Could you check a few things on this model? Use its own coordinates, in mm. A direction names the side the tool comes from. Coordinates: 2 decimals unless noted, no trailing zeros. Write each loop counter-clockwise with the first axis right and the second up, starting at its lowest first coordinate (ties: lowest second). Pieces come first, ordered by that corner, then holes. Notation, with made-up numbers: M 55,-15.75 L 102,-15.75 A21 cw 102,12.25 Z; hole C 29,8 d7. An arc over 180 degrees is marked long. Write item = value, one per line.
```python
from build123d import *

# Parameters (mm, degrees)
IZIM2_R                     = 5
Y_KSEKLIK_EKSTR_ZYON2_DEPTH = 21.5
IZIM2_5_R                   = 7.5
IZIM2_5_R_2                 = 5
Y_KSEKLIK_EKSTR_ZYON3_DEPTH = 16.5
IZIM18_R                    = 10
Y_KSEKLIK_EKSTR_ZYON6_DEPTH = 7.5
IZIM3_R                     = 7.5
Y_KSEKLIK_EKSTR_ZYON4_DEPTH = 50
S_P_R4_PROFILE_R            = 7.5
IZIM42_R                    = 5
KES_EKSTR_ZYON5_DEPTH       = 10
IZIM43_R                    = 5
Y_KSEKLIK_EKSTR_ZYON7_DEPTH = 15
IZIM44_R                    = 2.5
Y_KSEKLIK_EKSTR_ZYON8_DEPTH = 15


with BuildPart() as part:
    # izim2 → Y_kseklik-Ekstr_zyon2 (new, symmetric)
    with BuildSketch(Plane(origin=(0, 0, 0), x_dir=(1, 0, 0), z_dir=(0, 1, 0))):
        with Locations(Location((0, 0, 0), (0, 0, 270))):
            Circle(IZIM2_R)
    extrude(amount=Y_KSEKLIK_EKSTR_ZYON2_DEPTH, both=True)

    # izim2_5 → Y_kseklik-Ekstr_zyon3 (add, symmetric)
    with BuildSketch(Plane(origin=(0, 0, 0), x_dir=(1, 0, 0), z_dir=(0, 1, 0))):
        with Locations(Location((0, 0, 0), (0, 0, 270))):
            Circle(IZIM2_5_R)
        with Locations(Location((0, 0, 0), (0, 0, 270))):
            Circle(IZIM2_5_R_2, mode=Mode.SUBTRACT)
    extrude(amount=Y_KSEKLIK_EKSTR_ZYON3_DEPTH, both=True)

    # izim18 → Y_kseklik-Ekstr_zyon6 (add, symmetric)
    with BuildSketch(Plane(origin=(0, 0, 0), x_dir=(1, 0, 0), z_dir=(0, 1, 0))):
        with Locations(Location((0, 0, 0), (0, 0, 270))):
            Circle(IZIM18_R)
    extrude(amount=Y_KSEKLIK_EKSTR_ZYON6_DEPTH, both=True)

    # izim3 → Y_kseklik-Ekstr_zyon4 (add)
    with BuildSketch(Plane.XY):
        with Locations(Location((0, 0, 0), (0, 0, 90))):
            Circle(IZIM3_R)
    extrude(amount=Y_KSEKLIK_EKSTR_ZYON4_DEPTH)

    # S_p_r4: sweep along a path in izim22
    with BuildLine(Plane.XY) as s_p_r4_path:
        Line((0, 0), (17.792695878, 0))
        Line((17.792695878, 0), (58.393051363, 34.067743313))
    # S_p_r4 profile (on start of the path) → S_p_r4 (sweep)
    with BuildSketch(Plane(origin=(0, 0, 0), x_dir=(0, 0, 1), z_dir=(1, 0, 0))):
        Circle(S_P_R4_PROFILE_R)
    sweep(path=s_p_r4_path.line, transition=Transition.RIGHT)

    # izim42 → Kes-Ekstr_zyon5 (cut, symmetric)
    with BuildSketch(Plane(origin=(5.513634999, -6.570894318, -4.952333559), x_dir=(0.8267965189633342, 0.3839166530668254, 0.411114971422934), z_dir=(-0.5566703992264205, 0.6634139481689367, 0.500000000000001))):
        with Locations(Location((52.788286905, 21.97481992, 0), (0, 0, 208.340774423))):
            Circle(IZIM42_R)
    extrude(amount=KES_EKSTR_ZYON5_DEPTH, both=True, mode=Mode.SUBTRACT)

    # izim43 → Y_kseklik-Ekstr_zyon7 (add)
    with BuildSketch(Plane.XY.offset(50)):
        Circle(IZIM43_R)
    extrude(amount=Y_KSEKLIK_EKSTR_ZYON7_DEPTH)

    # izim44 → Y_kseklik-Ekstr_zyon8 (add)
    with BuildSketch(Plane.XY.offset(65)):
        Circle(IZIM44_R)
    extrude(amount=Y_KSEKLIK_EKSTR_ZYON8_DEPTH)


solid = part.part
```
Item 1: Imagine slicing it at B-B (z = 39). Write out the boundary of the cut face in (x, y).
Numbers:
outline = C 0,0 d15
Item 2: Imagine slicing it at A-A (z = 59). Write out the boundary of the cut face in (x, y), and give its area (3 significant figures).
Numbers:
outline = C 0,0 d10
area = 78.5 mm²
Item 3: If I drill on line 1 along Z through (x, y) = (48, 27); line 2 along Z through (x, y) = (4, 8); line 3 along Z through (x, y) = (-2, 11), over which ranges is the centre line in solid material (lowest first)?
Numbers:
line_1 = -7.39 to -4.08, 5.54 to 7.39
line_2 = -6.34 to 6.34
line_3 = -7.23 to 7.23
Item 4: I'm going to push flat-ended pins straight in: P1, Ø16, axis at x = -1, z = 3.5, coming from the +Y side; P2, Ø12, axis at x = 8.5, z = 19, coming from the -Y side; P3, Ø8, axis at y = 5.5, z = 11, coming from the -X side. Where does each tip first touch, or does it pass through?
Numbers:
P1 = 21.5
P2 = -7.07
P3 = -7.35
Item 5: If we mould it in two halves opening along X, with no side actions, what happens to faces 5 (the face through (58.46, 33.99, 0.11)), 6 (the face through (7, 7.5, 4)), 7 (the face through (0.33, -11.937, -7.493))? For each: pulls with the +X half, pulls with the -X half, needs draft (parallel to the pull), parting line crosses it, or undercut.
Numbers:
face_5 = pulls with the +X half
face_6 = undercut
face_7 = parting line crosses it
Item 6: For faces 1 (the face through (-7.436, -0.976, 28.003)), 2 (the face through (-5, 16.5, 2)), 3 (the face through (7.045, -5.914, 7.097)), 4 (the face through (-5, -16.5, 2)), which set-ups out of +Z, -Z, +X, -X, +Y, -Y let a thin tool reach every point of the face, with its end or its side?
Numbers:
face_1 = +Z
face_2 = +Y
face_3 = +Z, +X, -Y
face_4 = -Y
